The model under review builds one solid part; all positions refer to its coordinate system, in mm. Face numbers are marked on the shaded views. A direction names the side the tool comes from. Coordinates: 2 decimals unless noted, no trailing zeros. Order: outer loops, then holes, each group sorted by start corner. A loop starts at its lowest first (then second) coordinate and runs counter-clockwise, first axis right, second up.
Autodesk Inventor part; units mm, degrees
ref_plane "YZ Plane" through (0, 0, 0) normal (1, 0, 0) x (0, 1, 0)
ref_plane "XZ Plane" through (0, 0, 0) normal (0, 1, 0) x (-1, 0, 0)
ref_plane "XY Plane" through (0, 0, 0) normal (0, 0, 1) x (1, 0, 0)
sketch "Sketch1" plane through (0, 0, 0) normal (0, 1, 0) x (-1, 0, 0)
  circle A0 centre (0, 0) radius 116.3878
  circle A1 centre (0, 0) radius 126.3878
  line L0 (129.8416, -11.9217) -> (-129.8416, -11.9217)
  line L1 (125.8243, -171.9217) -> (-125.8243, -171.9217)
  circle A2 centre (0, 0) radius 130.3878
  circle A3 centre (0, 0) radius 25
  point P0 (-115.7756, -11.9217)
  point P1 (115.7756, -11.9217)
  point P2 (-125.8243, -11.9217)
  point P3 (125.8243, -11.9217)
  point P4 (-21.9744, -11.9217)
  point P5 (21.9744, -11.9217)
  dimension "d1" = 232.7756
  dimension "d2" = 10
  dimension "d6" = 160
  dimension "d7" = 171.9217
  dimension "d11" = 4
  dimension "d13" = 50
extrude "Extrusion1" add sketch "Sketch1" along normal blind 40 contours A0 L0 A3 | A0 L0 A1 | A3 L0 | L0 A2 A1 picked at (-80.805, 28.5699) picked at (-122.0572, 13.8082) picked at (7.5455, -2.0688) picked at (1.8738, 127.5443)
ref_plane "Work Plane2" through (0, 37, 0) normal (0, 1, 0) x (1, 0, 0)
ref_plane "Work Plane3" through (0, 3, 0) normal (0, -1, 0) x (1, 0, 0)
extrude "Extrusion2" cut sketch "Sketch1" along normal up to surface (34 mm away) from surface at 3 contours A0 L0 A3 | A0 L0 A1 | A3 L0 picked at (-80.805, 28.5699) picked at (-122.0572, 13.8082) picked at (7.5455, -2.0688)
extrude "Extrusion3" cut sketch "Sketch1" along normal up to surface (3 mm away) contours A3 L0 picked at (7.5455, -2.0688)
equation "\"d1\" = ballInletWheel_diameter"
equation "\"d2\" = ballInletWheel_margin"
equation "\"d6\" = profile_height"
equation "\"d3\" = profile_width"
equation "\"d14\" = profile_width"
equation "\"d8\" = -profileTallWall_thickness"
equation "\"d12\" = -profileTallWall_thickness"
properties part number "ballInletCover"
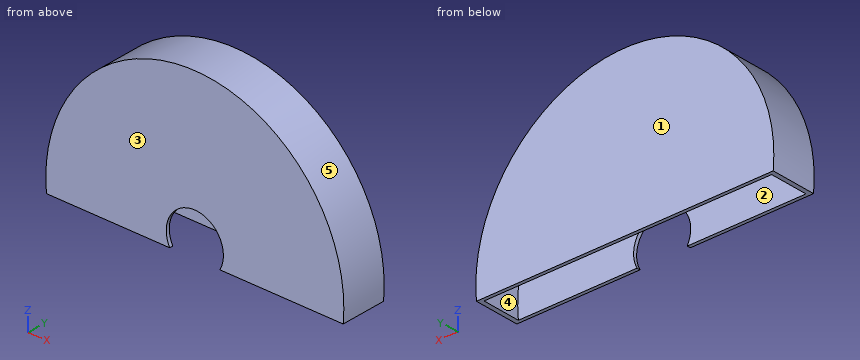
(1) We need section B-B, the plane x = 0. Write out the cut boundary in (y, z).
A:
outline: (0, 25) - (3, 25) - (3, 126.39) - (37, 126.39) - (37, -11.92) - (40, -11.92) - (40, 130.39) - (0, 130.39) - close
(2) For pin 1 Ø1.5 at (y, z) = (26.5, 41.5) entering from -X; pin 2 Ø4 at (y, z) = (29, 52) entering from +X; pin 3 Ø6 at (y, z) = (20.5, 73) entering from +X, all flat-tipped, find the tip position at first contact; note any pin that passes through.
A:
pin 1: stops at x = -123.86
pin 2: stops at x = 120.42
pin 3: stops at x = 110
(3) Wall thickness on probe 1 along X at (y, z) = (20, 0); probe 2 along Y at (x, z) = (37.5, 85); probe 3 along X at (y, z) = (32, 111): over which ranges is each line inside the solid? List them lowest first.
A:
probe 1: x = -130.39 to -126.39, 126.39 to 130.39
probe 2: y = 0 to 3, 37 to 40
probe 3: x = -68.41 to -60.44, 60.44 to 68.41
(4) Draft analysis for pull direction X (two halves, no side actions). For the marked faces 3, 4 and 5, state which applies: released by +X, released by -X, zero draft, split by the parting line, or undercut.
A:
face 3: zero draft
face 4: undercut
face 5: split by the parting line
(5) Machinability: for the marked faces 1 and 2, which of the approach directions +Z, -Z, +X, -X, +Y, -Y give a long, thin tool a straight path to every point of the face, cutting with its end or side? Answer none if there is none.
A:
face 1: +Z, -Z, +X, -X, +Y
face 2: -Z
(6) We need section C-C, the plane z = 0. Write out the cut boundary in (x, y).
A:
outline: (-130.39, 0) - (-25, 0) - (-25, 3) - (-126.39, 3) - (-126.39, 37) - (126.39, 37) - (126.39, 3) - (25, 3) - (25, 0) - (130.39, 0) - (130.39, 40) - (-130.39, 40) - close
(7) We need section A-A, the plane z = 64.5. Write out the cut boundary in (x, y).
A:
outline: (-113.32, 0) - (113.32, 0) - (113.32, 40) - (-113.32, 40) - close; hole (-108.69, 3) - (108.69, 3) - (108.69, 37) - (-108.69, 37) - close
(8) We need section D-D, the plane y = 30.5. Write out the cut boundary in (x, z), and give its area (3 significant figures).
A:
outline: (-129.84, -11.92) - (-125.82, -11.92) arc R126.39 cw (long way) to (125.82, -11.92) - (129.84, -11.92) arc R130.39 ccw (long way) to start
area: 1,710 mm2
